Autodesk Inventor part; units mm, degrees
ref_plane "Work Plane1" through (0, -10.9985, 10.795) normal (1, 0, 0) x (0, 0, -1)
ref_plane "YZ Plane" through (0, 0, 0) normal (1, 0, 0) x (0, 1, 0)
ref_plane "XZ Plane" through (0, 0, 0) normal (0, 1, 0) x (-1, 0, 0)
sketch "Sketch1" plane through (0, 0, 0) normal (0, 0, 1) x (1, 0, 0)
  arc A0 (-1.508, 2.794) -> (-1.508, -2.794) centre (0, 0) ccw
  line L0 (-3.175, 0) -> (0, 0) construction
  line L1 (0, 0) -> (3.175, 0) construction
  line L2 (-1.508, 2.794) -> (1.508, 2.794)
  line L3 (-1.508, -2.794) -> (1.508, -2.794)
  arc A1 (1.508, 2.794) -> (-1.508, 2.794) centre (0, 0) ccw construction
  arc A2 (1.508, -2.794) -> (1.508, 2.794) centre (0, 0) ccw
  arc A3 (-1.508, -2.794) -> (1.508, -2.794) centre (0, 0) ccw construction
  circle A4 centre (0, 0) radius 3.429 construction
  circle A5 centre (0, 0) radius 4.064
  circle A6 centre (0, 0) radius 12.7
  dimension "d1" = 2.794
  dimension "d2" = 3.175
  dimension "d3" = 6.858
  dimension "d5" = 0.635
  dimension "d6" = 25.4
extrude "Extrusion1" add sketch "Sketch1" along normal blind 3.048 contours A5 | A6
sketch "Sketch2" plane through (0, 0, 3.048) normal (0, 0, 1) x (1, 0, 0)
  circle A0 centre (0, 0) radius 12.7
  arc A1 (-1.508, 2.794) -> (-1.508, -2.794) centre (0, 0) ccw
extrude "Extrusion2" add sketch "Sketch2" along normal blind 3.175
hole "Hole1" at (0, 0, 3.048) direction (0, 0, 1) diameter 3.302 depth 25.4 tip angle 118
sketch "Sketch3" plane through (0, 0, 6.223) normal (0, 0, 1) x (1, 0, 0)
  circle A0 centre (0, 0) radius 12.7
  circle A1 centre (0, 0) radius 3.429
  circle A2 centre (0, 0) radius 4.064
  dimension "d18" = 6.858
  dimension "d19" = 0.635
extrude "Extrusion3" add sketch "Sketch3" along normal blind 4.572 contours A0
sketch "Sketch4" plane through (0, 0, 10.795) normal (0, 0, 1) x (1, 0, 0)
  circle A0 centre (0, 0) radius 4.064
  circle A1 centre (0, 0) radius 12.7
  line L0 (-6.35, 10.9985) -> (-6.35, -10.9985)
  line L1 (0, 12.7) -> (0, -12.7)
  line L2 (6.35, 10.9985) -> (6.35, -10.9985)
  line L3 (-9.525, 8.4003) -> (-9.525, -8.4003)
  line L4 (9.525, 8.4003) -> (9.525, -8.4003)
  dimension "d22" = 6.35
  dimension "d23" = 3.175
extrude "Extrusion4" add sketch "Sketch4" along normal blind 7.9375 contours A1 L4 L2 | L0 A1 L3
sketch "Sketch5" plane through (-6.35, -10.9985, 10.795) normal (1, 0, 0) x (0, 0, -1)
  line L0 (0, 21.997) -> (0, 0)
  line L1 (0, 21.997) -> (-7.9375, 21.997)
  line L2 (-7.9375, 0) -> (-7.9375, 21.997)
  line L3 (0, 0) -> (-7.9375, 0)
  line L4 (-3.9688, 21.997) -> (-3.9688, 0) construction
  line L5 (-7.9375, 10.9985) -> (0, 10.9985) construction
  line L6 (-7.9375, 16.4978) -> (0, 16.4978) construction
  line L7 (-7.9375, 5.4993) -> (0, 5.4993) construction
  point P0 (10.795, 10.9985)
  point P1 (-3.9688, 16.4978)
  point P2 (-3.9688, 5.4993)
  dimension "d26" = 5.4993
  dimension "d27" = 5.4993
hole "Hole2" at (-6.35, 5.4993, 14.7638) at (-6.35, -5.4993, 14.7638) direction (-1, 0, 0) diameter 3.302 end through all
ref_plane "Work Plane1" through (0, -10.9985, 10.795) normal (1, 0, 0) x (0, 0, -1)
mirror "Mirror1" about plane through (0, -10.9985, 10.795) normal (1, 0, 0) of "Hole2"
equation "\"d26\" = d27"
properties part number "Pneumatic Connector -Actuator Side"
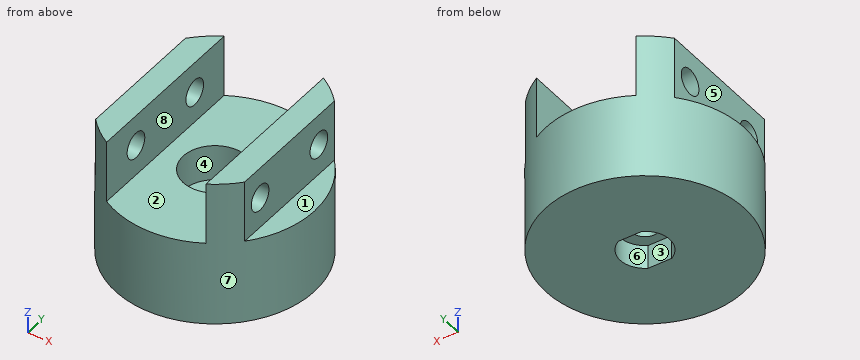
The model under review builds one solid part; all positions refer to its coordinate system, in mm. Face numbers are marked on the shaded views. A direction names the side the tool comes from. Give positions to 0.01 mm unless a question says otherwise; leave off trailing zeros. Write each loop counter-clockwise with the first axis right and the second up, starting at its lowest first coordinate (ties: lowest second). Pieces come first, ordered by that corner, then holes.
1. Add section A-A, the plane x = 0. Write out the cut boundary in (y, z) (3 decimals).
2. Tool access review of the marked faces 1, 2, 3, 4 and 5: name each direction out of +Z, -Z, +X, -X, +Y, -Y from which nothing blocks a thin tool from reaching the whole face with its end or side.
3. Draft analysis for pull direction Y (two halves, no side actions). For the marked faces 6, 7 and 8, state which applies: +Y half, -Y half, draft (parallel to the pull), parting line (faces both ways), or undercut.
4. For P1, Ø2.5, axis at y = 5.5, z = 14.76, coming from the -X side; P2, Ø5, axis at y = -8, z = 5, coming from the +X side; P3, Ø6.5, axis at y = 5.5, z = 15.5, coming from the -X side (3 decimals); P4, Ø6, axis at x = 6.5, z = 11, coming from the -Y side, all flat-tipped, find the tip position at first contact; note any pin that passes through.
5. Wall thickness on L1, parallel to Y at x = 0, z = 10; L2, parallel to X at y = -3.5, z = 12.5 (3 decimals); L3, parallel to Z at x = -3.5, y = -11.25 (3 decimals): over which ranges is each line inside the solid? List them lowest first.
Worked answers:
1. outline: (-12.7, 0) - (-2.794, 0) - (-2.794, 3.048) - (-1.651, 3.048) - (-1.651, 6.223) - (-4.064, 6.223) - (-4.064, 10.795) - (-12.7, 10.795) - close; (1.651, 3.048) - (2.794, 3.048) - (2.794, 0) - (12.7, 0) - (12.7, 10.795) - (4.064, 10.795) - (4.064, 6.223) - (1.651, 6.223) - close
2. face 1: +Z, +X, +Y, -Y
2. face 2: +Z, +Y, -Y
2. face 3: -Z
2. face 4: +Z
2. face 5: +Z, -X, +Y, -Y
3. face 6: undercut
3. face 7: parting line
3. face 8: draft
4. P1: passes through
4. P2: stops at x = 11.45
4. P3: stops at x = -9.525
4. P4: stops at y = -12.21
5. L1: y = -12.7 to -4.06, 4.06 to 12.7
5. L2: x = -9.525 to -6.35, 6.35 to 9.525
5. L3: z = 0 to 10.795
